```python
from build123d import *

# Parameters (mm, degrees)
SKETCH1_W             = 25
SKETCH1_H             = 83.4
BOSS_EXTRUDE1_DEPTH   = 2
SKETCH2_W             = 11.6
SKETCH2_H             = 11.6
SKETCH2_W_2           = 12
SKETCH2_H_2           = 12
BOSS_EXTRUDE2_DEPTH   = 2
CHAMFER1_SIZE         = 11.3
CHAMFER1_SIZE2        = 1.992494882
CHAMFER1_PART_2_SIZE  = 11.3
CHAMFER1_PART_2_SIZE2 = 1.992494882
SKETCH4_W             = 5
SKETCH4_H             = 81.4
BOSS_EXTRUDE3_DEPTH   = 3


with BuildPart() as part:
    # Sketch1 → Boss-Extrude1 (new body)
    with BuildSketch(Plane(origin=(0, 0, 0), x_dir=(1, 0, 0), z_dir=(0, 1, 0))):
        with Locations((12.5, 41.7)):
            Rectangle(SKETCH1_W, SKETCH1_H)
    extrude(amount=BOSS_EXTRUDE1_DEPTH)

    # Sketch2 → Boss-Extrude2 (add)
    with BuildSketch(Plane(origin=(0, 2, 0), x_dir=(1, 0, 0), z_dir=(0, 1, 0))):
        with Locations((5.8, -0.2)):
            Rectangle(SKETCH2_W, SKETCH2_H)
        with Locations((2, 81.4)):
            Rectangle(SKETCH2_W_2, SKETCH2_H_2)
    extrude(amount=BOSS_EXTRUDE2_DEPTH)

    # Chamfer1
    chamfer1_edges = [part.edges().sort_by_distance(p)[0] for p in [
        (5.8, 4, -5.6),
    ]]
    chamfer1_side = [part.faces().sort_by_distance(p)[0] for p in [
        (5.8, 4, 0.2),
    ]]
    chamfer(chamfer1_edges, length=CHAMFER1_SIZE, length2=CHAMFER1_SIZE2, reference=chamfer1_side[0])

    # Chamfer1 part 2
    chamfer1_part_2_edges = [part.edges().sort_by_distance(p)[0] for p in [
        (8, 4, -81.4),
        (2, 4, -75.4),
    ]]
    chamfer1_part_2_side = [part.faces().sort_by_distance(p)[0] for p in [
        (2, 4, -81.4),
    ]]
    chamfer(chamfer1_part_2_edges, length=CHAMFER1_PART_2_SIZE, length2=CHAMFER1_PART_2_SIZE2, reference=chamfer1_part_2_side[0])

    # Sketch4 → Boss-Extrude3 (add)
    with BuildSketch(Plane.XZ):
        with Locations((22.5, -40.7)):
            Rectangle(SKETCH4_W, SKETCH4_H)
    extrude(amount=BOSS_EXTRUDE3_DEPTH)


solid = part.part
```
Input: part model. Units: mm. Frame: model coordinates. A direction names the side the tool comes from. Round coordinates to 2 decimals unless told otherwise and drop trailing zeros. Order: outer loops, then holes, each group sorted by start corner. A loop starts at its lowest first (then second) coordinate and runs counter-clockwise, first axis right, second up. Notation, with made-up numbers: (-25, 37.25) - (-11, 37.25) arc R14 ccw to (-11, 60.25) - close; hole circle Ø2 at (37.5, 64.5). An arc over 180 degrees is marked (long way). One line per question, with ' | ' between items. Start each with the question number.
1) Cut plane C-C, the plane y = 1. Return the cut outline in (x, z).
2) Ray query, probe 1 along Y at (x, z) = (16, -74); probe 2 along X at (y, z) = (-2.5, -28.5); probe 3 along Z at (x, y) = (3, 1). Return the intervals inside material, ascending.
3) Set-up query: faces 1 (the flat face through (11.6, 3, 2)), 2 (the flat face through (20, -1, -41)), 3 (the flat face through (22, -1, -81.4)), 4 (the flat face through (3.68, 2.77, -82.65)), 5 (the flat face through (0.58, 2.77, -79.72)). Return all of +Z, -Z, +X, -X, +Y, -Y with unobstructed straight access to the full face (end or side cutting, diameter ignored); none if empty.
4) Contact query for flat-ended pins moving along their axis: P1, Ø1.6, axis at x = 12.5, y = 1.5, coming from the -Z side; P2, Ø0.6, axis at y = 3.5, z = 1.5, coming from the +X side; P3, Ø2.5, axis at y = -1, z = -54, coming from the -X side. Output: stop coordinate, or through.
5) Cut plane B-B, the plane z = -50.5. Return the cut outline in (x, y).
6) Pull-direction query (Z, two-part tool) for faces 6 (the flat face through (0, 1, -38)), 7 (the flat face through (1, 3, -87.4)), 8 (the flat face through (12, 2, -42)); classes: +Z half, -Z half, draft (parallel to the pull), parting line (faces both ways), or undercut.
Worked out:
1) outline: (0, -83.4) - (25, -83.4) - (25, 0) - (0, 0) - close
2) probe 1: y = 0 to 2 | probe 2: x = 20 to 25 | probe 3: z = -83.4 to 0
3) face 1: +Z, -Z, +X, +Y | face 2: +Z, -Z, -X, -Y | face 3: -Z, +X, -X, -Y | face 4: -Z, +X, +Y | face 5: +X, -X, +Y
4) P1: stops at z = -83.4 | P2: stops at x = 11.6 | P3: stops at x = 0
5) outline: (0, 0) - (20, 0) - (20, -3) - (25, -3) - (25, 2) - (0, 2) - close
6) face 6: draft | face 7: -Z half | face 8: undercut
